Check sheet for the modelled part. Datum: model origin and axes. Units: mm. A direction names the side the tool comes from. Give positions to 0.01 mm unless a question says otherwise; leave off trailing zeros. Write each loop counter-clockwise with the first axis right and the second up, starting at its lowest first coordinate (ties: lowest second). Pieces come first, ordered by that corner, then holes. Notation, with made-up numbers: M 42.25,82.25 L 65.25,82.25 A35 ccw 65.25,115.25 Z; hole C 22.5,61.25 d5. An arc over 180 degrees is marked long. Write item = value, one per line. Start each with the question number.
1) Cross-section at B-B, the plane z = 9.5. Record the cut outline in (x, y), plus the area to 3 significant figures.
2) Cross-section at A-A, the plane y = -6. Record the cut outline in (x, z), plus the area to 3 significant figures.
3) Mould release check, pull along Y, two halves, no side actions. Record for faces 1 (the flat face through (26, -28, -1)), 2 (the flat face through (26, -29, -2.5)), 3 (the cylindrical face through (59.972, -13.852, 13.792)): released by +Y, released by -Y, zero draft, split by the parting line, or undercut.
4) Cross-section at C-C, the plane x = 16. Record the cut outline in (y, z).
5) Go/stop test with flat-tipped pins: pin 1 (2.5 mm diameter, centred on y = -10.5, z = 10, fed in from +X); pin 2 (4.5 mm diameter, centred on x = 55.5, z = 10.5, fed in from -Y); pin 3 (1.5 mm diameter, centred on x = 20.5, y = -27, fed in from -Z). Record where each tip stops, or that it passes through.
6) Scan lines: line 1 along Y through (x, z) = (58.25, 9.5); line 2 along Y through (x, z) = (28.5, 1); line 3 along X through (y, z) = (-25.75, 2.25). Record each from-to range of solid material in increasing order. Write a range as [from, to].
7) Access from +Z, -Z, +X, -X, +Y, -Y to the whole of each face (thin tool, end or side, straight path). Record for faces 4 (the flat face through (55, -17, 5.4)), 5 (the cylindrical face through (13.88, -22.43, 0.99)), 6 (the flat face through (55, -12.1, 10)).
8) Cross-section at D-D, the plane y = -21.75. Record the cut outline in (x, z), plus the area to 3 significant figures.
```python
from build123d import *

# Parameters (mm, degrees)
SKETCH1_W           = 52
SKETCH1_H           = 30
BOSS_EXTRUDE1_DEPTH = 2
SKETCH2_W           = 4
SKETCH2_H           = 30
BOSS_EXTRUDE2_DEPTH = 20
FILLET1_R           = 3
SKETCH4_R           = 1.725
CUT_EXTRUDE2_DEPTH  = 2
SKETCH5_W           = 51.988371154
SKETCH5_H           = 2
BOSS_EXTRUDE3_DEPTH = 2.5
SKETCH6_W           = 20
SKETCH6_H           = 14
CUT_EXTRUDE3_DEPTH  = 2
SKETCH7_W           = 8.2
SKETCH7_H           = 5.8
SKETCH7_W_2         = 5.8
SKETCH7_H_2         = 3.4
BOSS_EXTRUDE4_DEPTH = 6
SKETCH8_R           = 5.5
SKETCH8_R_2         = 4.25
BOSS_EXTRUDE5_DEPTH = 6
SKETCH10_R          = 4.5
SKETCH10_R_2        = 3.7
BOSS_EXTRUDE6_DEPTH = 10
FILLET2_R           = 2


with BuildPart() as part:
    # Sketch1 → Boss-Extrude1 (new body)
    with BuildSketch(Plane.XY):
        with Locations((26, -15)):
            Rectangle(SKETCH1_W, SKETCH1_H)
    extrude(amount=BOSS_EXTRUDE1_DEPTH)

    # Sketch2 → Boss-Extrude2 (add)
    with BuildSketch(Plane(origin=(0, 0, 2), x_dir=(-1, 0, 0), z_dir=(0, 0, -1))):
        with Locations((-50, -15)):
            Rectangle(SKETCH2_W, SKETCH2_H)
    extrude(amount=-BOSS_EXTRUDE2_DEPTH)

    # Fillet1
    fillet1_edges = [part.edges().sort_by_distance(p)[0] for p in [
        (50, -30, 22),
        (50, 0, 22),
    ]]
    fillet(fillet1_edges, radius=FILLET1_R)

    # Sketch4 → Cut-Extrude2 (cut)
    with BuildSketch(Plane.XY.offset(2)):
        with Locations((41.277695867, -6)):
            Circle(SKETCH4_R)
        with Locations((6.277695867, -6)):
            Circle(SKETCH4_R)
    extrude(amount=-CUT_EXTRUDE2_DEPTH, mode=Mode.SUBTRACT)

    # Sketch5 → Boss-Extrude3 (add)
    with BuildSketch(Plane(origin=(0, 0, 0), x_dir=(-1, 0, 0), z_dir=(0, 0, -1))):
        with Locations((-25.994185577, -29)):
            Rectangle(SKETCH5_W, SKETCH5_H)
        Polygon((-52, -1.965960074), (0, -2.193486325), (0, 0), (-52, 0), align=None)
    extrude(amount=BOSS_EXTRUDE3_DEPTH)

    # Sketch6 → Cut-Extrude3 (cut)
    with BuildSketch(Plane.XY.offset(2)):
        with Locations((23.277695867, -16)):
            Rectangle(SKETCH6_W, SKETCH6_H)
    extrude(amount=-CUT_EXTRUDE3_DEPTH, mode=Mode.SUBTRACT)

    # Sketch7 → Boss-Extrude4 (add)
    with BuildSketch(Plane(origin=(52, 0, 0), x_dir=(0, 0, -1), z_dir=(1, 0, 0))):
        with Locations((-9.5, -15)):
            Rectangle(SKETCH7_W, SKETCH7_H)
        with Locations((-9.5, -15)):
            Rectangle(SKETCH7_W_2, SKETCH7_H_2, mode=Mode.SUBTRACT)
    extrude(amount=BOSS_EXTRUDE4_DEPTH)

    # Sketch8 → Boss-Extrude5 (add)
    with BuildSketch(Plane(origin=(52, 0, 0), x_dir=(0, 0, -1), z_dir=(1, 0, 0))):
        with Locations((-9.5, -12.5)):
            Circle(SKETCH8_R)
        with Locations((-9.5, -12.5)):
            Circle(SKETCH8_R_2, mode=Mode.SUBTRACT)
    extrude(amount=BOSS_EXTRUDE5_DEPTH)

    # Sketch10 → Boss-Extrude6 (add)
    with BuildSketch(Plane(origin=(52, 0, 0), x_dir=(0, 0, -1), z_dir=(1, 0, 0))):
        with Locations(Location((-9.5, -12.5, 0), (0, 0, 180))):
            Circle(SKETCH10_R)
        with Locations(Location((-9.5, -12.5, 0), (0, 0, 173.793732249))):
            Circle(SKETCH10_R_2, mode=Mode.SUBTRACT)
    extrude(amount=BOSS_EXTRUDE6_DEPTH)

    # Fillet2
    fillet2_edges = [part.edges().sort_by_distance(p)[0] for p in [
        (33.277695867, -9, 1),
        (33.277695867, -23, 1),
        (13.277695867, -23, 1),
        (13.277695867, -9, 1),
    ]]
    fillet(fillet2_edges, radius=FILLET2_R)


solid = part.part
```
Reply:
q1.outline = M 48,-30 L 52,-30 L 52,-18 L 58,-18 L 58,-17 L 62,-17 L 62,-16.2 L 52,-16.2 L 52,-13.3 L 58,-13.3 L 58,-12.1 L 52,-12.1 L 52,-8.8 L 62,-8.8 L 62,-8 L 58,-8 L 58,-7 L 52,-7 L 52,0 L 48,0 Z
q1.area = 155 mm2
q2.outline = M 0,0 L 4.55,0 L 4.55,2 L 0,2 Z; M 8,0 L 39.55,0 L 39.55,2 L 8,2 Z; M 43,0 L 52,0 L 52,22 L 48,22 L 48,2 L 43,2 Z
q2.area = 170 mm2
q3.face_1 = undercut
q3.face_2 = zero draft
q3.face_3 = split by the parting line
q4.outline = M -30,-2.5 L -28,-2.5 L -28,0 L -23,0 L -23,2 L -30,2 Z; M -9,0 L -2.12,0 L -2.12,-2.5 L 0,-2.5 L 0,2 L -9,2 Z
q5.pin_1 = 52
q5.pin_2 = -18
q5.pin_3 = 0
q6.line_1 = [-17, -16.2], [-8.8, -8]
q6.line_2 = [-30, -23], [-9, 0]
q6.line_3 = [48, 52]
q7.face_4 = -Z, +X, -Y
q7.face_5 = +Z, -Z
q7.face_6 = +X
q8.outline = M 0,0 L 13.42,0 L 13.42,2 L 0,2 Z; M 33.13,0 L 52,0 L 52,22 L 48,22 L 48,2 L 33.13,2 Z
q8.area = 145 mm2
